Verification items for the finished model (mm, model axes). Face numbers are marked on the shaded views. A direction names the side the tool comes from. Give positions to 0.01 mm unless a question says otherwise; leave off trailing zeros. Loops run counter-clockwise (first coordinate to the right, second up) from the corner with the lowest first, then second, coordinate; pieces in that order, holes last. Notation, with made-up numbers: (29.5, 52) - (34.5, 52) arc R24 ccw to (34.5, 91) - close; hole circle Ø3 at (71.5, 81). An arc over 180 degrees is marked (long way). Use one line per item in the form item = value.
```python
from build123d import *

# Parameters (mm, degrees)
SKETCH1_R           = 5.08
SKETCH1_R_2         = 1.4605
BOSS_EXTRUDE1_DEPTH = 3.175
FILLET1_R           = 2.54
SKETCH2_W           = 2.54
SKETCH2_H           = 3.175
BOSS_EXTRUDE2_DEPTH = 1.27


with BuildPart() as part:
    # Sketch1 → Boss-Extrude1 (new body)
    with BuildSketch(Plane(origin=(0, 0, 0), x_dir=(1, 0, 0), z_dir=(0, 1, 0))):
        Circle(SKETCH1_R)
        Circle(SKETCH1_R_2, mode=Mode.SUBTRACT)
        with BuildLine():
            Line((40.720655575, 4.445), (2.459344425, 4.445))
            ThreePointArc((2.459344425, 4.445), (4.376063852, 2.580012628), (5.08, 0))
            ThreePointArc((5.08, 0), (4.376063852, -2.580012628), (2.459344425, -4.445))
            Line((2.459344425, -4.445), (40.720655575, -4.445))
            ThreePointArc((40.720655575, -4.445), (38.1, 0), (40.720655575, 4.445))
        make_face()
        with Locations((43.18, 0)):
            Circle(SKETCH1_R)
        with Locations((43.18, 0)):
            Circle(SKETCH1_R_2, mode=Mode.SUBTRACT)
    extrude(amount=BOSS_EXTRUDE1_DEPTH)

    # Fillet1
    fillet1_edges = [part.edges().sort_by_distance(p)[0] for p in [
        (2.459344425, 1.5875, -4.445),
        (40.720655575, 1.5875, -4.445),
        (40.720655575, 1.5875, 4.445),
        (2.459344425, 1.5875, 4.445),
    ]]
    fillet(fillet1_edges, radius=FILLET1_R)

    # Sketch2 → Boss-Extrude2 (add)
    with BuildSketch(Plane.XY.offset(4.445)):
        with Locations((26.67, 1.5875)):
            Rectangle(SKETCH2_W, SKETCH2_H)
        with Locations((21.59, 1.5875)):
            Rectangle(SKETCH2_W, SKETCH2_H)
    extrude(amount=BOSS_EXTRUDE2_DEPTH)


solid = part.part
```
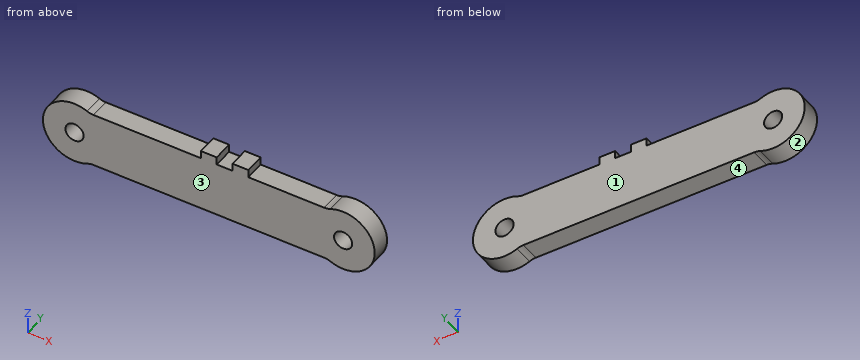
1. Section check A-A, the plane z = 0. Record the cut outline in (x, y) (1 decimal), then the cut area to 3 significant figures.
Result set:
outline = (-5.1, 0) - (-1.5, 0) - (-1.5, 3.2) - (-5.1, 3.2) - close; (1.5, 0) - (41.7, 0) - (41.7, 3.2) - (1.5, 3.2) - close; (44.6, 0) - (48.3, 0) - (48.3, 3.2) - (44.6, 3.2) - close
area = 151 mm²
2. Tool access check on the marked faces 3 and 4. Record the directions out of +Z, -Z, +X, -X, +Y, -Y that give a thin tool (end or side, any length) a straight path to the whole face; none if there is none.
Result set:
face_3 = +Z, -Z, +X, -X, -Y
face_4 = -Z, +Y, -Y
3. Section check B-B, the plane y = 1.6. Record the cut outline in (x, z) (1 decimal).
Result set:
outline = (2, -4.7) arc R2.5 cw to (3, -4.4) - (40.1, -4.4) arc R2.5 cw to (41.1, -4.7) arc R5.1 ccw (long way) to (41.1, 4.7) arc R2.5 cw to (40.1, 4.4) - (27.9, 4.4) - (27.9, 5.7) - (25.4, 5.7) - (25.4, 4.4) - (22.9, 4.4) - (22.9, 5.7) - (20.3, 5.7) - (20.3, 4.4) - (3, 4.4) arc R2.5 cw to (2, 4.7) arc R5.1 ccw (long way) to start; hole circle Ø2.9 at (0, 0); hole circle Ø2.9 at (43.2, 0)
4. Section check C-C, the plane x = 43.18. Record the cut outline in (y, z) (1 decimal), then the cut area to 3 significant figures.
Result set:
outline = (0, -5.1) - (3.2, -5.1) - (3.2, -1.5) - (0, -1.5) - close; (0, 1.5) - (3.2, 1.5) - (3.2, 5.1) - (0, 5.1) - close
area = 23.0 mm²
5. Draft check along X on the marked faces 1 and 2. Enter one of: released by +X, released by -X, zero draft, split by the parting line, or undercut.
Result set:
face_1 = zero draft
face_2 = undercut
6. Section check D-D, the plane x = 34. Record the cut outline in (y, z) (3 decimals).
Result set:
outline = (0, -4.445) - (3.175, -4.445) - (3.175, 4.445) - (0, 4.445) - close
7. Scan lines: probe 1 along X at (y, z) = (1.4, 0); probe 2 along Z at (x, y) = (43.18, 1.3); probe 3 along X at (y, z) = (0.4, -1.25). Record each from-to range of solid material in increasing order.
Result set:
probe_1 = -5.08 to -1.46, 1.46 to 41.72, 44.64 to 48.26
probe_2 = -5.08 to -1.46, 1.46 to 5.08
probe_3 = -4.92 to -0.76, 0.76 to 42.42, 43.94 to 48.1
8. Depth check by flat-ended pin: pin 1 Ø1 at (y, z) = (1, 5) entering from +X; pin 2 Ø1.6 at (x, y) = (16.5, 1) entering from -Z (3 decimals); pin 3 Ø0.6 at (y, z) = (1.5, 5.5) entering from -X. Enter the tip coordinate at first touch or a pass-through.
Result set:
pin_1 = 45.54
pin_2 = -4.445
pin_3 = 20.32
